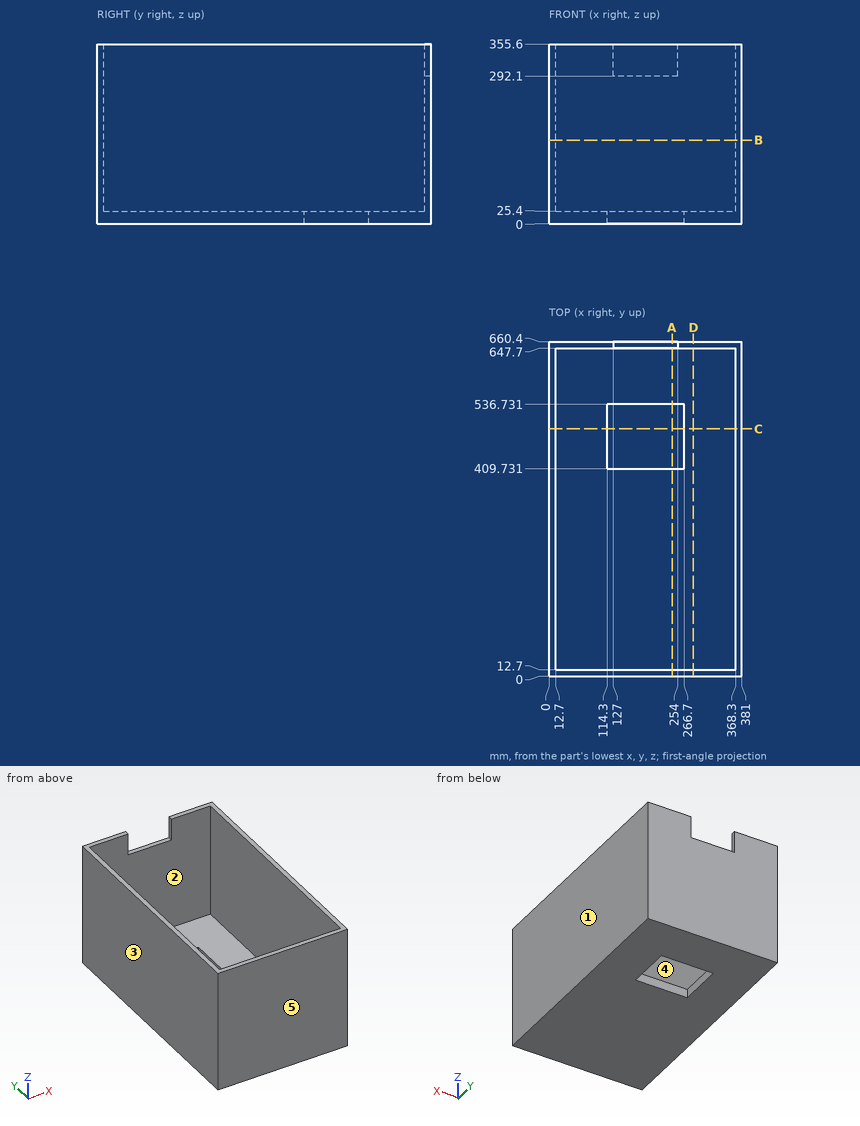
Geometry check sheet. Reference: drawing and pictorial views, mm from the part's lowest x, y, z. A direction names the side the tool comes from. Round coordinates to 2 decimals unless told otherwise and drop trailing zeros. Order: outer loops, then holes, each group sorted by start corner. A loop starts at its lowest first (then second) coordinate and runs counter-clockwise, first axis right, second up.
Q1. Cross-section at C-C, the plane y = 488.5. Enter the section's corners in (x, z).
Filled sheet:
outline: (0, 0) - (114.3, 0) - (114.3, 25.4) - (12.7, 25.4) - (12.7, 355.6) - (0, 355.6) - close; (266.7, 0) - (381, 0) - (381, 355.6) - (368.3, 355.6) - (368.3, 25.4) - (266.7, 25.4) - close
Q2. Set-up check for the marked faces 1 and 2: record each of +Z, -Z, +X, -X, +Y, -Y from which the full face is reachable in a straight line by a thin tool's end or side.
Filled sheet:
face 1: +Z, -Z, +X, +Y, -Y
face 2: +Z
Q3. Cross-section at A-A, the plane x = 243. Enter the section's corners in (y, z).
Filled sheet:
outline: (0, 0) - (409.73, 0) - (409.73, 25.4) - (12.7, 25.4) - (12.7, 355.6) - (0, 355.6) - close; (536.73, 0) - (660.4, 0) - (660.4, 292.1) - (647.7, 292.1) - (647.7, 25.4) - (536.73, 25.4) - close
Q4. Cross-section at B-B, the plane z = 165.5. Enter the section's corners in (x, y), plus the area to 3 significant figures.
Filled sheet:
outline: (0, 0) - (381, 0) - (381, 660.4) - (0, 660.4) - close; hole (12.7, 12.7) - (368.3, 12.7) - (368.3, 647.7) - (12.7, 647.7) - close
area: 25,800 mm2
Q5. Depth check by flat-ended pin: P1, Ø4, axis at x = 189, y = 657, coming from the +Z side. Enter the tip coordinate at first touch or a pass-through.
Filled sheet:
P1: stops at z = 292.1
Q6. Scan lines: L1, parallel to Y at x = 133.5, z = 136; L2, parallel to X at y = 331, z = 177; L3, parallel to Y at x = 152.5, z = 22. Record each from-to range of solid material in increasing order.
Filled sheet:
L1: y = 0 to 12.7, 647.7 to 660.4
L2: x = 0 to 12.7, 368.3 to 381
L3: y = 0 to 409.73, 536.73 to 660.4
Q7. Cross-section at D-D, the plane x = 285. Enter the section's corners in (y, z), plus the area to 3 significant figures.
Filled sheet:
outline: (0, 0) - (660.4, 0) - (660.4, 355.6) - (647.7, 355.6) - (647.7, 25.4) - (12.7, 25.4) - (12.7, 355.6) - (0, 355.6) - close
area: 25,200 mm2
Q8. Draft check along Y on the marked faces 3, 4 and 5. Enter one of: pulls with the +Y half, pulls with the -Y half, needs draft (parallel to the pull), parting line crosses it, or undercut.
Filled sheet:
face 3: needs draft
face 4: undercut
face 5: pulls with the -Y half
